Model file for the job. Use its own axes, mm. Give positions to 0.01 mm unless a question says otherwise; leave off trailing zeros. Write each loop counter-clockwise with the first axis right and the second up, starting at its lowest first coordinate (ties: lowest second). Pieces come first, ordered by that corner, then holes.
```python
from build123d import *

# Parameters (mm, degrees)
SKETCH2_R           = 7.25
SKETCH2_R_2         = 2.25
BOSS_EXTRUDE1_DEPTH = 6
CUT_EXTRUDE1_START  = -6
CUT_EXTRUDE1_DEPTH  = 6


with BuildPart() as part:
    # Sketch2 → Boss-Extrude1 (new body)
    with BuildSketch(Plane(origin=(0, 0, 0), x_dir=(1, 0, 0), z_dir=(0, 1, 0))):
        with BuildLine():
            Line((-16.25, 90), (-16.25, -90))
            ThreePointArc((-16.25, -90), (0, -106.25), (16.25, -90))
            Line((16.25, -90), (16.25, 90))
            ThreePointArc((16.25, 90), (0, 106.25), (-16.25, 90))
        make_face()
        with Locations(Location((0, 90, 0), (0, 0, 270))):
            Circle(SKETCH2_R, mode=Mode.SUBTRACT)
        with Locations(Location((0, -90, 0), (0, 0, 270))):
            Circle(SKETCH2_R, mode=Mode.SUBTRACT)
        with Locations(Location((8, 98, 0), (0, 0, 270))):
            Circle(SKETCH2_R_2, mode=Mode.SUBTRACT)
        with Locations(Location((-8, 98, 0), (0, 0, 270))):
            Circle(SKETCH2_R_2, mode=Mode.SUBTRACT)
        with Locations(Location((-8, 82, 0), (0, 0, 270))):
            Circle(SKETCH2_R_2, mode=Mode.SUBTRACT)
        with Locations(Location((8, 82, 0), (0, 0, 270))):
            Circle(SKETCH2_R_2, mode=Mode.SUBTRACT)
        with Locations(Location((8, -98, 0), (0, 0, 90))):
            Circle(SKETCH2_R_2, mode=Mode.SUBTRACT)
        with Locations(Location((8, -82, 0), (0, 0, 90))):
            Circle(SKETCH2_R_2, mode=Mode.SUBTRACT)
        with Locations(Location((-8, -82, 0), (0, 0, 90))):
            Circle(SKETCH2_R_2, mode=Mode.SUBTRACT)
        with Locations(Location((-8, -98, 0), (0, 0, 90))):
            Circle(SKETCH2_R_2, mode=Mode.SUBTRACT)
        with Locations(Location((0, 50.402785483, 0), (0, 0, 270))):
            Circle(SKETCH2_R, mode=Mode.SUBTRACT)
        with Locations(Location((0, -38.452553576, 0), (0, 0, 270))):
            Circle(SKETCH2_R_2, mode=Mode.SUBTRACT)
    extrude(amount=BOSS_EXTRUDE1_DEPTH)

    # Sketch3 → Cut-Extrude1 (cut)
    with BuildSketch(Plane(origin=(0, 6, 0), x_dir=(1, 0, 0), z_dir=(0, 1, 0)).offset(CUT_EXTRUDE1_START)):
        Polygon((-12.25, 30.324358358), (-2, 20.074358358), (-2, -9.624126451), (-12.25, 0.625873549), align=None)
        Polygon((-12.25, -5.030980701), (-12.25, -23.874126451), (-2.828427125, -14.452553576), align=None)
        Polygon((-9.421572875, 33.152785483), (-2, 33.152785483), (-2, 25.731212608), align=None)
        Polygon((12.25, -23.874126451), (2.828427125, -14.452553576), (12.25, -5.030980701), align=None)
        Polygon((9.421572875, 33.152785483), (2, 33.152785483), (2, 25.731212608), align=None)
        Polygon((2, -9.624126451), (12.25, 0.625873549), (12.25, 30.324358358), (2, 20.074358358), align=None)
        Polygon((-12.25, 71.336551667), (-2, 61.086551667), (-2, 71.75), align=None)
        with BuildLine():
            Line((-12.25, 65.679697418), (-12.25, 55.452537952))
            ThreePointArc((-12.25, 55.452537952), (-10.391208444, 58.623812614), (-7.732662193, 61.162359611))
            Line((-7.732662193, 61.162359611), (-12.25, 65.679697418))
        make_face()
        with BuildLine():
            Line((-12.25, 41.179697418), (-12.25, 37.152785483))
            Line((-12.25, 37.152785483), (-2, 37.152785483))
            Line((-2, 37.152785483), (-2, 37.304598586))
            ThreePointArc((-2, 37.304598586), (-6.92090289, 39.103953544), (-10.759574128, 42.67012329))
            Line((-10.759574128, 42.67012329), (-12.25, 41.179697418))
        make_face()
        with BuildLine():
            Line((12.25, 41.179697418), (12.25, 37.152785483))
            Line((12.25, 37.152785483), (2, 37.152785483))
            Line((2, 37.152785483), (2, 37.304598586))
            ThreePointArc((2, 37.304598586), (6.92090289, 39.103953544), (10.759574128, 42.67012329))
            Line((10.759574128, 42.67012329), (12.25, 41.179697418))
        make_face()
        with BuildLine():
            Line((12.25, 65.679697418), (7.732662193, 61.162359611))
            ThreePointArc((7.732662193, 61.162359611), (10.391208444, 58.623812614), (12.25, 55.452537952))
            Line((12.25, 55.452537952), (12.25, 65.679697418))
        make_face()
        Polygon((2, 61.086551667), (2, 71.75), (12.25, 71.336551667), align=None)
        with BuildLine():
            Line((-2, -19.280980701), (-12.25, -29.530980701))
            Line((-12.25, -29.530980701), (-12.25, -34.729465511))
            Line((-12.25, -34.729465511), (-2, -44.979465511))
            Line((-2, -44.979465511), (-2, -43.306675536))
            ThreePointArc((-2, -43.306675536), (-5.25, -38.452553576), (-2, -33.598431616))
            Line((-2, -33.598431616), (-2, -19.280980701))
        make_face()
        Polygon((-12.25, -40.38631976), (-12.25, -59.229465511), (-2.828427125, -49.807892635), align=None)
        with BuildLine():
            Line((-2, -54.63631976), (-12.25, -64.88631976))
            Line((-12.25, -64.88631976), (-12.25, -79.322921748))
            ThreePointArc((-12.25, -79.322921748), (-7.628207354, -75.651726495), (-2, -73.873546577))
            Line((-2, -73.873546577), (-2, -54.63631976))
        make_face()
        with BuildLine():
            Line((12.25, -64.88631976), (12.25, -79.322921748))
            ThreePointArc((12.25, -79.322921748), (7.628207354, -75.651726495), (2, -73.873546577))
            Line((2, -73.873546577), (2, -54.63631976))
            Line((2, -54.63631976), (12.25, -64.88631976))
        make_face()
        Polygon((12.25, -59.229465511), (2.828427125, -49.807892635), (12.25, -40.38631976), align=None)
        with BuildLine():
            Line((12.25, -34.729465511), (2, -44.979465511))
            Line((2, -44.979465511), (2, -43.306675536))
            ThreePointArc((2, -43.306675536), (5.25, -38.452553576), (2, -33.598431616))
            Line((2, -33.598431616), (2, -19.280980701))
            Line((2, -19.280980701), (12.25, -29.530980701))
            Line((12.25, -29.530980701), (12.25, -34.729465511))
        make_face()
    extrude(amount=CUT_EXTRUDE1_DEPTH, mode=Mode.SUBTRACT)


solid = part.part
```
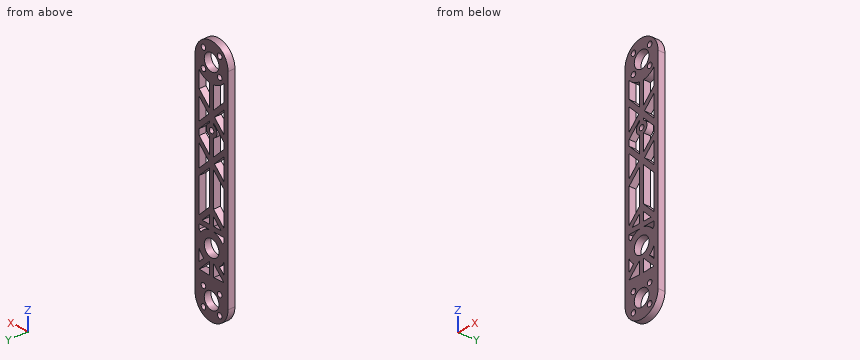
1. Pin check, flat tips, straight feed: P1, Ø3.5, axis at x = -8, z = 82, coming from the +Y side; P2, Ø3, axis at x = -10.5, y = 2.5, coming from the -Z side; P3, Ø1, axis at x = -12.5, y = 3, coming from the +Z side; P4, Ø1.5, axis at x = 7.5, y = 1, coming from the +Z side. Stop position of each tip, or through.
Calculated:
P1: passes through
P2: stops at z = -103.53
P3: stops at z = 100.96
P4: stops at z = 104.78
2. Probe probe 1 along X at (y, z) = (2.45, -82); probe 2 along X at (y, z) = (5.35, -65); probe 3 along X at (y, z) = (0.3, 15). List the from-to ranges inside material, lowest first.
Calculated:
probe 1: x = -16.25 to -10.25, -5.75 to 5.75, 10.25 to 16.25
probe 2: x = -16.25 to -12.25, -11.57 to -5.91, -2 to 2, 5.91 to 11.57, 12.25 to 16.25
probe 3: x = -16.25 to -12.25, -3.38 to 3.38, 12.25 to 16.25
3. Slice it at C-C, the plane z = -11. Write the cut outline in (x, y), and give its area (3 significant figures).
Calculated:
outline: (-16.25, 0) - (-12.25, 0) - (-12.25, 6) - (-16.25, 6) - close; (-2, 0) - (2, 0) - (2, 6) - (-2, 6) - close; (12.25, 0) - (16.25, 0) - (16.25, 6) - (12.25, 6) - close
area: 72.0 mm2
4. Slice it at B-B, the plane z = 52.5. Write the cut outline in (x, y), and give its area (3 significant figures).
Calculated:
outline: (-16.25, 0) - (-12.25, 0) - (-12.25, 6) - (-16.25, 6) - close; (-5.52, 0) - (5.52, 0) - (5.52, 6) - (-5.52, 6) - close; (12.25, 0) - (16.25, 0) - (16.25, 6) - (12.25, 6) - close
area: 114 mm2
5. Slice it at A-A, the plane x = 0. Write the cut outline in (y, z).
Calculated:
outline: (0, -106.25) - (6, -106.25) - (6, -97.25) - (0, -97.25) - close; (0, -82.75) - (6, -82.75) - (6, -57.65) - (0, -57.65) - close; (0, -43.15) - (6, -43.15) - (6, 36.2) - (0, 36.2) - close; (0, 40.7) - (6, 40.7) - (6, 82.75) - (0, 82.75) - close; (0, 97.25) - (6, 97.25) - (6, 106.25) - (0, 106.25) - close
6. Slice it at D-D, the plane y = 2.5. State how many separate pieces and enclosed holes the cut face has, and give its area (3 significant figures).
Calculated:
separate pieces: 1
enclosed holes: 30
area: 4,220 mm2
